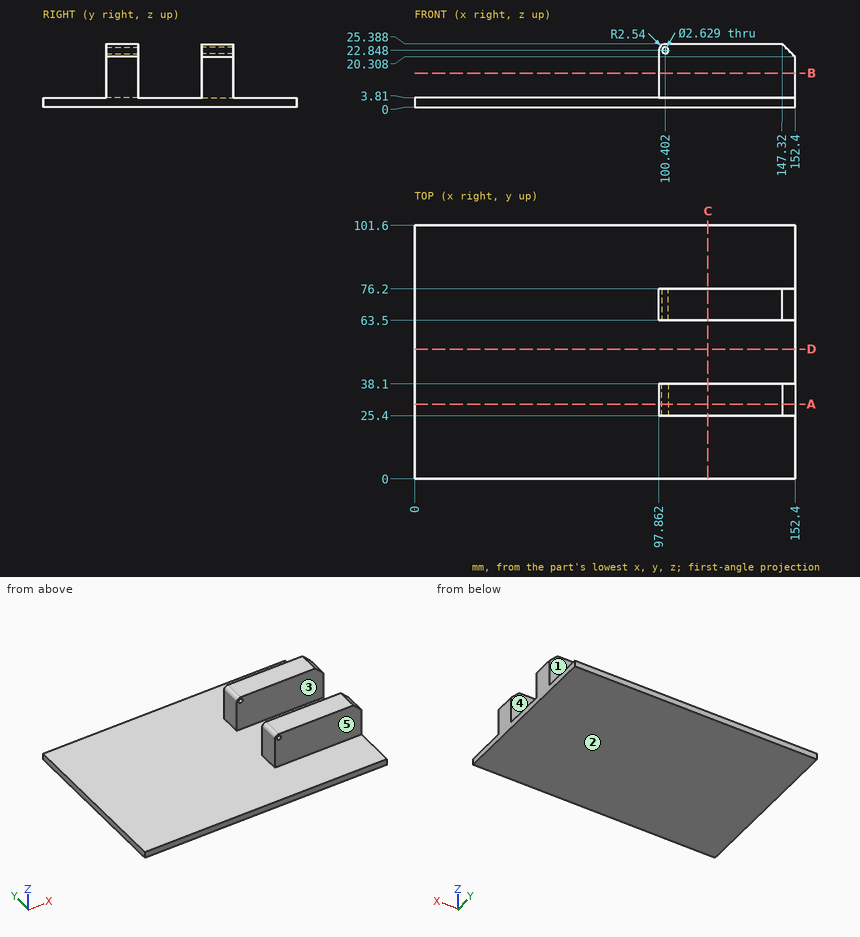
Study the drawing (mm; zero at the part's minimum x, y, z) and answer. A direction names the side the tool comes from. Coordinates: 2 decimals unless noted, no trailing zeros. Loops run counter-clockwise (first coordinate to the right, second up) from the corner with the lowest first, then second, coordinate; pieces in that order, holes last. Notation, with made-up numbers: M 67,21 L 90,21 A14 ccw 90,40 Z; hole C 34,-8 d4. An arc over 180 degrees is marked long. Answer in a Markdown table with one row per item.
1) Find section D-D (y = 52). Determine the outline of the cut face in (x, z).
Answers below:
| item | result |
|---|---|
| outline | M 0,0 L 152.4,0 L 152.4,3.81 L 0,3.81 Z |
2) Which of the six approach directions +Z, -Z, +X, -X, +Y, -Y give full straight-line access (tool end or side, diameter ignored) to the marked faces 4 and 5?
Answers below:
| item | result |
|---|---|
| face 4 | +Z, +X, -X |
| face 5 | +Z, +X, -X, -Y |
3) Find section C-C (x = 117.5). Determine the outline of the cut face in (y, z), then the cut area to 3 significant figures.
Answers below:
| item | result |
|---|---|
| outline | M 0,0 L 101.6,0 L 101.6,3.81 L 76.2,3.81 L 76.2,25.39 L 63.5,25.39 L 63.5,3.81 L 38.1,3.81 L 38.1,25.39 L 25.4,25.39 L 25.4,3.81 L 0,3.81 Z |
| area | 935 mm^2 |
4) Find section B-B (z = 13.75). Determine the outline of the cut face in (x, y).
Answers below:
| item | result |
|---|---|
| outline | M 97.86,25.4 L 152.4,25.4 L 152.4,38.1 L 97.86,38.1 Z; M 97.86,63.5 L 152.4,63.5 L 152.4,76.2 L 97.86,76.2 Z |
5) Find the intervals of material crossed by probe 1 along Y at (x, z) = (109.5, 11); probe 2 along Z at (x, y) = (112, 11); probe 3 along X at (y, z) = (70.5, 14.5), in increasing order.
Answers below:
| item | result |
|---|---|
| probe 1 | 25.4 to 38.1, 63.5 to 76.2 |
| probe 2 | 0 to 3.81 |
| probe 3 | 97.86 to 152.4 |
6) Given pin 1 (14 mm diameter, centred on y = 69.5, z = 17, fed in from -X); pin 2 (4 mm diameter, centred on x = 94, y = 36.5, fed in from +Z); pin 3 (5 mm diameter, centred on y = 78, z = 11, fed in from +X); pin 4 (3 mm diameter, centred on x = 100.4, z = 22.85, fed in from -Y), each flat-ended and moving along its own axis, determine where each tip first touches the part or whether it passes through.
Answers below:
| item | result |
|---|---|
| pin 1 | x = 97.86 |
| pin 2 | z = 3.81 |
| pin 3 | x = 152.4 |
| pin 4 | y = 25.4 |
7) Determine the mould class of the marked faces 1, 2 and 3 for opening direction Y: released by +Y, released by -Y, zero draft, split by the parting line, or undercut.
Answers below:
| item | result |
|---|---|
| face 1 | released by +Y |
| face 2 | zero draft |
| face 3 | undercut |
8) Find section A-A (y = 30). Determine the outline of the cut face in (x, z) (1 decimal), then the cut area to 3 significant figures.
Answers below:
| item | result |
|---|---|
| outline | M 0,0 L 152.4,0 L 152.4,20.3 L 147.3,25.4 L 100.4,25.4 A2.5 ccw 97.9,22.8 L 97.9,3.8 L 0,3.8 Z; hole C 100.4,22.8 d2.6 |
| area | 1,740 mm^2 |
